Geometry check sheet. Reference: the model listing, model coordinates, mm. Give positions to 0.01 mm unless a question says otherwise; leave off trailing zeros. Loops run counter-clockwise (first coordinate to the right, second up) from the corner with the lowest first, then second, coordinate; pieces in that order, holes last.
```python
from build123d import *

# Parameters (mm, degrees)
F0_W     = 112.4385967851
F0_H     = 188.8671554625
F0_R     = 15.875
F0_R_2   = 12.7
F0_R_3   = 19.05
F1_DEPTH = 3.175
F2_W     = 112.4385967851
F2_H     = 188.8671554625
F3_DEPTH = 25.4


with BuildPart() as f1:
    # F0 (on Top) → F1 (new body)
    with BuildSketch(Plane.XY):
        with Locations((28.6107622087, 28.6107677966)):
            Rectangle(F0_W, F0_H)
        with Locations((-3.1392377913, -31.75)):
            Circle(F0_R, mode=Mode.SUBTRACT)
        with Locations((28.6107622087, -28.6004)):
            Circle(F0_R_2, mode=Mode.SUBTRACT)
        Circle(F0_R_2, mode=Mode.SUBTRACT)
        with Locations((28.6107622087, 0)):
            Circle(F0_R_2, mode=Mode.SUBTRACT)
        with Locations((60.3607622087, -31.75)):
            Circle(F0_R, mode=Mode.SUBTRACT)
        with Locations((57.2215244174, 0)):
            Circle(F0_R_2, mode=Mode.SUBTRACT)
        with Locations((0, 28.6107677966)):
            Circle(F0_R_2, mode=Mode.SUBTRACT)
        with Locations((0, 57.2111677966)):
            Circle(F0_R_2, mode=Mode.SUBTRACT)
        with Locations((28.6107622087, 28.6107677966)):
            Circle(F0_R_2, mode=Mode.SUBTRACT)
        with Locations((28.6107622087, 57.2111677966)):
            Circle(F0_R_2, mode=Mode.SUBTRACT)
        with Locations((28.6107622087, 95.3111677966)):
            Circle(F0_R_3, mode=Mode.SUBTRACT)
        with Locations((57.2215244174, 28.6107677966)):
            Circle(F0_R_2, mode=Mode.SUBTRACT)
        with Locations((57.2215244174, 57.2111677966)):
            Circle(F0_R_2, mode=Mode.SUBTRACT)
    extrude(amount=F1_DEPTH)

    # F2 (on face) → F3 (cut)
    with BuildSketch(Plane.XY.offset(3.175)):
        with Locations((28.6107622087, 28.6107677966)):
            Rectangle(F2_W, F2_H)
        with BuildLine():
            ThreePointArc((20.8784768956, 71.1167105009), (13.6314439157, 115.824091125), (54.0107622087, 95.3111677966))
            ThreePointArc((54.0107622087, 95.3111677966), (49.1236855371, 80.3318495036), (36.3430475218, 71.1167105009))
            ThreePointArc((36.3430475218, 71.1167105009), (40.1631717397, 68.1516517023), (42.9161433131, 64.1759668261))
            ThreePointArc((42.9161433131, 64.1759668261), (60.7952365635, 72.715390949), (73.1322866261, 57.2111677966))
            ThreePointArc((73.1322866261, 57.2111677966), (70.7147963313, 48.7800369638), (64.1969551584, 42.9109677966))
            ThreePointArc((64.1969551584, 42.9109677966), (70.7147963313, 37.0418986294), (73.1322866261, 28.6107677966))
            ThreePointArc((73.1322866261, 28.6107677966), (70.7116620279, 20.1746228647), (64.1863240909, 14.3053870058))
            ThreePointArc((64.1863240909, 14.3053870058), (70.7116660444, 8.4361490481), (73.132292214, 0))
            ThreePointArc((73.132292214, 0), (71.2000982328, -7.5994740585), (65.8728052171, -13.3531970855))
            ThreePointArc((65.8728052171, -13.3531970855), (75.766649881, -20.2833701277), (79.5655786775, -31.75))
            ThreePointArc((79.5655786775, -31.75), (63.1358397408, -50.7532607805), (41.9579378153, -37.2419058575))
            ThreePointArc((41.9579378153, -37.2419058575), (28.6107622087, -44.5008), (15.2635866021, -37.2419058575))
            ThreePointArc((15.2635866021, -37.2419058575), (-16.7116606729, -45.3372849651), (-8.6512807997, -13.3531970855))
            ThreePointArc((-8.6512807997, -13.3531970855), (-15.8808701583, 0.9749332764), (-6.9529550782, 14.3111476674))
            ThreePointArc((-6.9529550782, 14.3111476674), (-15.9003988973, 28.6048460855), (-6.9636042292, 42.9052050468))
            ThreePointArc((-6.9636042292, 42.9052050468), (-11.2510776635, 68.4613058168), (14.3053811044, 64.1759668261))
            ThreePointArc((14.3053811044, 64.1759668261), (17.0583526777, 68.1516517023), (20.8784768956, 71.1167105009))
        make_face(mode=Mode.SUBTRACT)
        with BuildLine():
            ThreePointArc((14.3053811043, -6.9648117949), (10.8191046051, -11.6661693551), (5.8687746425, -14.7888476926))
            ThreePointArc((5.8687746425, -14.7888476926), (10.4436598742, -18.1731864338), (13.8259486181, -22.7495874708))
            ThreePointArc((13.8259486181, -22.7495874708), (16.9457643394, -17.795283394), (21.6471515982, -14.3059658585))
            ThreePointArc((21.6471515982, -14.3059658585), (17.3606227479, -11.2510841251), (14.3053811044, -6.9648117949))
        make_face()
        with BuildLine():
            ThreePointArc((35.5743728192, -14.3059658585), (40.275760078, -17.795283394), (43.3955757993, -22.7495874708))
            ThreePointArc((43.3955757993, -22.7495874708), (46.7778645432, -18.1731864338), (51.352749775, -14.7888476926))
            ThreePointArc((51.352749775, -14.7888476926), (46.4024198123, -11.6661693551), (42.9161433131, -6.9648117949))
            ThreePointArc((42.9161433131, -6.9648117949), (39.8609016695, -11.2510841251), (35.5743728192, -14.3059658585))
        make_face()
        with BuildLine():
            ThreePointArc((14.2996204416, 21.6578133609), (11.2432809162, 17.3674873857), (6.9529550782, 14.3111476674))
            ThreePointArc((6.9529550782, 14.3111476674), (11.2459493597, 11.2552723147), (14.3053811043, 6.9648117949))
            ThreePointArc((14.3053811044, 6.9648117949), (17.3601551723, 11.2506165694), (21.6459625352, 14.3053870058))
            ThreePointArc((21.6459625352, 14.3053870058), (17.355498357, 17.3648178728), (14.2996204416, 21.6578133609))
        make_face()
        with BuildLine():
            ThreePointArc((50.2567247439, 14.3053870058), (45.9709163125, 17.3601601983), (42.9161433131, 21.6459687672))
            ThreePointArc((42.9161433131, 21.6459687672), (39.8613703136, 17.3601601983), (35.5755618822, 14.3053870058))
            ThreePointArc((35.5755618822, 14.3053870058), (39.8613692451, 11.2506165694), (42.9161433131, 6.9648117949))
            ThreePointArc((42.9161433131, 6.9648117949), (45.970917381, 11.2506165694), (50.2567247439, 14.3053870058))
        make_face()
        with BuildLine():
            ThreePointArc((21.6353314677, 42.9109677966), (17.3559736701, 45.9647421861), (14.3053811044, 50.2463687672))
            ThreePointArc((14.3053811044, 50.2463687672), (11.2501380202, 45.9600901332), (6.9636042292, 42.9052050468))
            ThreePointArc((6.9636042292, 42.9052050468), (11.2474674185, 39.8498601457), (14.2996204416, 35.5637222323))
            ThreePointArc((14.2996204416, 35.5637222323), (17.3513196546, 39.8525340027), (21.6353314677, 42.9109677966))
        make_face()
        with BuildLine():
            ThreePointArc((50.2460936764, 42.9109677966), (45.9667358788, 45.9647421861), (42.9161433131, 50.2463687672))
            ThreePointArc((42.9161433131, 50.2463687672), (39.8655507473, 45.9647421861), (35.5861929497, 42.9109677966))
            ThreePointArc((35.5861929497, 42.9109677966), (39.8655507473, 39.8571934072), (42.9161433131, 35.5755668261))
            ThreePointArc((42.9161433131, 35.5755668261), (45.9667358788, 39.8571934072), (50.2460936764, 42.9109677966))
        make_face()
    extrude(amount=-F3_DEPTH, mode=Mode.SUBTRACT)


solid = f1.part
```
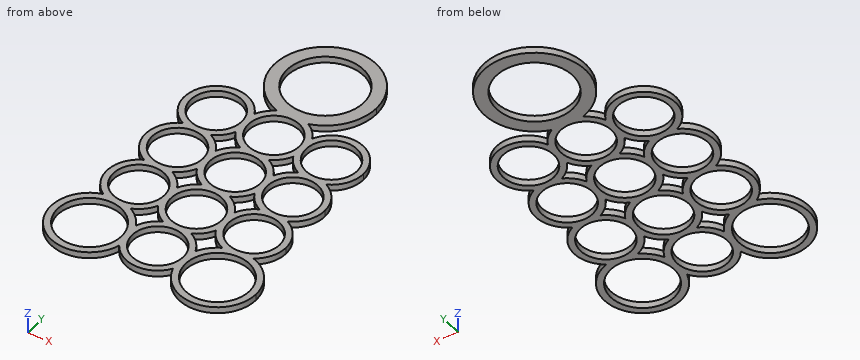
1) Sectioned sample at B-B on x = 0. Enter the section's corners in (y, z) (1 decimal).
2) Sectioned sample at D-D on z = 1. Count the separate pieces of the cut face and the enclosed holes in it, plus the area to 3 significant figures.
3) Depth check by flat-ended pin: P1, Ø1, axis at y = 5.5, z = 1.5, coming from the -X side; P2, Ø1, axis at x = 29, z = 0.5, coming from the -Y side; P3, Ø1, axis at y = 79, z = 2, coming from the -X side. Enter the tip coordinate at first touch or a pass-through.
4) Scan lines: line 1 along Y through (x, z) = (2, 2.65); line 2 along Y through (x, z) = (58, 2.55); line 3 along Y through (x, z) = (23.5, 1.4). Record each from-to range of solid material in increasing order.
5) Sectioned sample at C-C on x = 29.5. Enter the section's corners in (y, z) (3 decimals), plus the area to 3 significant figures.
6) Sectioned sample at A-A on y = 32. Enter the section's corners in (x, z) (3 decimals).
Determined:
1. outline: (-50.7, 0) - (-47.3, 0) - (-47.3, 3.2) - (-50.7, 3.2) - close; (-16.2, 0) - (-12.7, 0) - (-12.7, 3.2) - (-16.2, 3.2) - close; (12.7, 0) - (15.9, 0) - (15.9, 3.2) - (12.7, 3.2) - close; (41.3, 0) - (44.5, 0) - (44.5, 3.2) - (41.3, 3.2) - close; (69.9, 0) - (73.1, 0) - (73.1, 3.2) - (69.9, 3.2) - close
2. separate pieces: 1
2. enclosed holes: 19
2. area: 3,950 mm2
3. P1: stops at x = -15.1
3. P2: stops at y = -44.5
3. P3: stops at x = 8.73
4. line 1: y = -50.25 to -46.77, -16.73 to -12.54, 12.54 to 16.07, 41.15 to 44.67, 69.75 to 73
4. line 2: y = -50.81 to -47.45, -16.05 to -12.68, 12.68 to 15.93, 41.29 to 44.54, 69.89 to 73.1
4. line 3: y = -43.66 to -40.23, -16.97 to -11.63, 11.63 to 16.98, 40.24 to 45.58, 68.84 to 76.96, 113.66 to 120.19
5. outline: (-44.476, 0) - (-41.269, 0) - (-41.269, 3.175) - (-44.476, 3.175) - close; (-15.932, 0) - (-12.669, 0) - (-12.669, 3.175) - (-15.932, 3.175) - close; (12.669, 0) - (15.942, 0) - (15.942, 3.175) - (12.669, 3.175) - close; (41.28, 0) - (44.542, 0) - (44.542, 3.175) - (41.28, 3.175) - close; (69.88, 0) - (76.282, 0) - (76.282, 3.175) - (69.88, 3.175) - close; (114.34, 0) - (120.696, 0) - (120.696, 3.175) - (114.34, 3.175) - close
5. area: 81.8 mm2
6. outline: (-15.535, 0) - (-12.239, 0) - (-12.239, 3.175) - (-15.535, 3.175) - close; (12.239, 0) - (16.371, 0) - (16.371, 3.175) - (12.239, 3.175) - close; (40.85, 0) - (44.982, 0) - (44.982, 3.175) - (40.85, 3.175) - close; (69.461, 0) - (72.767, 0) - (72.767, 3.175) - (69.461, 3.175) - close
